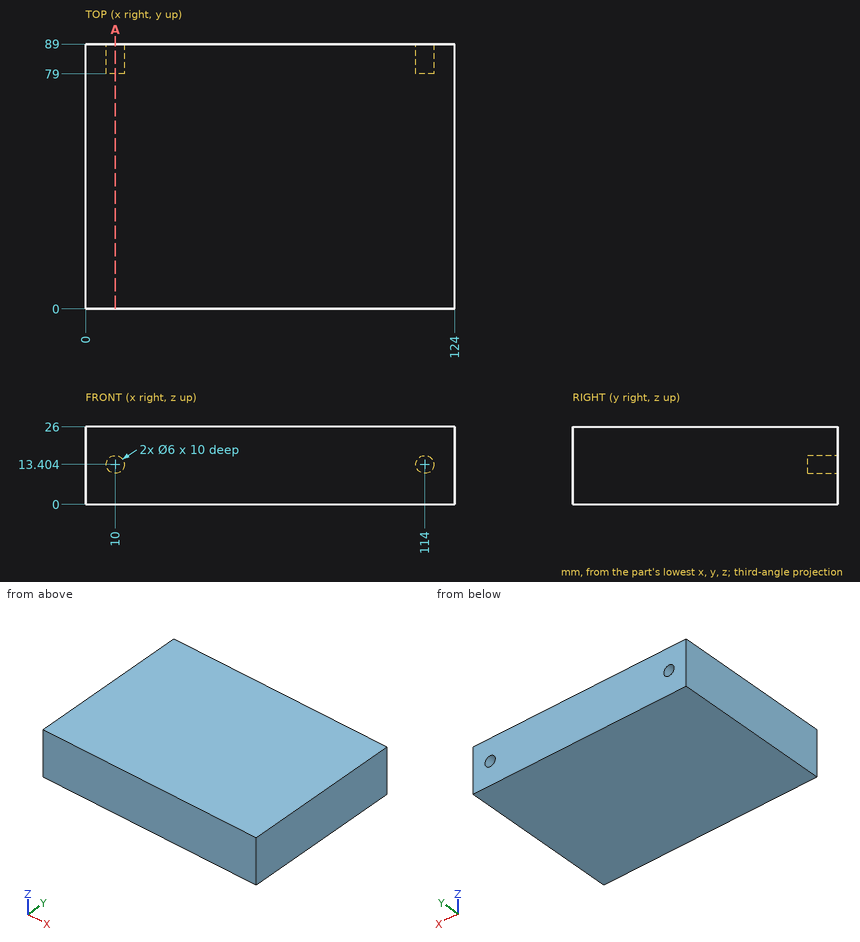
Part print with two shaded views. Sizes in mm from the minimum x, y, z corner. Round coordinates to 2 decimals unless told otherwise and drop trailing zeros. Loops run counter-clockwise (first coordinate to the right, second up) from the corner with the lowest first, then second, coordinate; pieces in that order, holes last.
Item 1: Pin check, flat tip, straight feed: P1, Ø1.8, axis at x = 10, z = 12.5, coming from the +Y side. Stop position of the tip, or through.
Item 2: Saw through at A-A (x = 10). List the corners of the cut face in (y, z), then the cut area to 3 significant figures.
Item 3: Drill centre lines: line 1 along Z through (x, y) = (10, 86); line 2 along Y through (x, z) = (114, 11). Where is each one in solid material? Low to high.
Worked answers:
1. P1: stops at y = 79
2. outline: (0, 0) - (89, 0) - (89, 10.4) - (79, 10.4) - (79, 16.4) - (89, 16.4) - (89, 26) - (0, 26) - close
2. area: 2,250 mm2
3. line 1: z = 0 to 10.4, 16.4 to 26
3. line 2: y = 0 to 79
